```python
from build123d import *

# Parameters (mm, degrees)
F1_DEPTH = 12
F2_R     = 3.5
F4_DEPTH = 4
F6_DEPTH = 4


with BuildPart() as f1:
    # F0 (on Top) → F1 (new body)
    with BuildSketch(Plane.XY):
        with BuildLine():
            Line((10.9868871146, 38.4103373848), (-46.3684160233, 38.4103373848))
            Line((-46.3684160233, 38.4103373848), (-44.9722234273, -1.5713874258))
            ThreePointArc((-44.9722234273, -1.5713874258), (-39.9691757058, -6.4027744503), (-34.9661279843, -1.5713874258))
            Line((-34.9661279843, -1.5713874258), (-36.0131128854, 28.4103373848))
            Line((-36.0131128854, 28.4103373848), (0.9868871146, 28.4103373848))
            Line((0.9868871146, 28.4103373848), (0.9868871146, -26.5896626152))
            ThreePointArc((0.9868871146, -26.5896626152), (35.472835987, -54.4539482888), (55.4723899987, -14.8848072183))
            ThreePointArc((55.4723899987, -14.8848072183), (48.8600464406, -12.3794304662), (46.3546696885, -18.9917740242))
            ThreePointArc((46.3546696885, -18.9917740242), (33.3725030493, -44.6770059472), (10.9868871146, -26.5896626152))
            Line((10.9868871146, -26.5896626152), (10.9868871146, 38.4103373848))
        make_face()
    extrude(amount=F1_DEPTH)

    # F2
    f2_edges = [f1.edges().sort_by_distance(p)[0] for p in [
        (10.986887, 38.410337, 6),
        (-46.368416, 38.410337, 6),
    ]]
    fillet(f2_edges, radius=F2_R)

    # F3 (on face) → F4 (cut)
    with BuildSketch(Plane.XY.offset(12)):
        with BuildLine():
            Line((7.4868871146, 35.16033604), (-42.744059925, 35.16033604))
            ThreePointArc((-42.744059925, 35.16033604), (-42.9238939077, 35.0840010432), (-42.9939062878, 34.9016125575))
            Line((-42.9939062878, 34.9016125575), (-41.7242018955, -1.4579640146))
            ThreePointArc((-41.7242018955, -1.4579640146), (-40.0114090798, -3.1522651845), (-38.219126663, -1.5422839975))
            Line((-38.219126663, -1.5422839975), (-39.3785877977, 31.6603387296))
            Line((-39.3785877977, 31.6603387296), (4.2368884594, 31.6603387296))
            Line((4.2368884594, 31.6603387296), (4.2368884594, -26.5896626152))
            ThreePointArc((4.2368884594, -26.5896626152), (34.7902274998, -51.276440713), (52.5091296718, -16.2195719825))
            ThreePointArc((52.5091296718, -16.2195719825), (50.1948112049, -15.3426907931), (49.3179300155, -17.65700926))
            ThreePointArc((49.3179300155, -17.65700926), (34.0551115365, -47.854513523), (7.7368857699, -26.5896626152))
            Line((7.7368857699, -26.5896626152), (7.7368857699, 34.9103373848))
            ThreePointArc((7.7368857699, 34.9103373848), (7.663662859, 35.0871131292), (7.4868871146, 35.16033604))
        make_face()
    extrude(amount=-F4_DEPTH, mode=Mode.SUBTRACT)

    # F5 (on face) → F6 (cut)
    with BuildSketch(Plane(origin=(0, 0, 0), x_dir=(1, 0, 0), z_dir=(0, 0, -1))):
        with BuildLine():
            Line((-41.7242032033, 1.4579640602), (-42.9939075956, -34.9016125119))
            ThreePointArc((-42.9939075956, -34.9016125119), (-42.923894849, -35.0840019523), (-42.744059925, -35.1603373486))
            Line((-42.744059925, -35.1603373486), (7.4868871146, -35.1603373486))
            ThreePointArc((7.4868871146, -35.1603373486), (7.6636637843, -35.0871140545), (7.7368870784, -34.9103373848))
            Line((7.7368870784, -34.9103373848), (7.7368870784, 26.5896626152))
            ThreePointArc((7.7368870784, 26.5896626152), (34.0551112616, 47.8545122436), (49.3179288223, 17.6570097974))
            ThreePointArc((49.3179288223, 17.6570097974), (50.1948106674, 15.3426896), (52.5091308649, 16.2195714451))
            ThreePointArc((52.5091308649, 16.2195714451), (34.7902277746, 51.2764419924), (4.2368871508, 26.5896626152))
            Line((4.2368871508, 26.5896626152), (4.2368871508, -31.660337421))
            Line((4.2368871508, -31.660337421), (-39.3785864427, -31.660337421))
            Line((-39.3785864427, -31.660337421), (-38.2191253525, 1.5422840291))
            ThreePointArc((-38.2191253525, 1.5422840291), (-40.0114090726, 3.1522664936), (-41.7242032033, 1.4579640602))
        make_face()
    extrude(amount=-F6_DEPTH, mode=Mode.SUBTRACT)


solid = f1.part
```
Check sheet for the modelled part. Datum: model origin and axes. Units: mm. A direction names the side the tool comes from. Coordinates: 2 decimals unless noted, no trailing zeros. Write each loop counter-clockwise with the first axis right and the second up, starting at its lowest first coordinate (ties: lowest second). Pieces come first, ordered by that corner, then holes. Notation, with made-up numbers: (-27, 27) -> (-23, 27) arc R36 cw to (-23, 61) -> close; hole circle Ø6 at (71.25, -10). An arc over 180 degrees is marked (long way). Use a Markdown table: item, result.
1. Sectioned sample at A-A (y = -20.5). Enter the section's corners in (x, z).
Reported:
| item | result |
|---|---|
| outline | (0.99, 0) -> (4.24, 0) -> (4.24, 4) -> (7.74, 4) -> (7.74, 0) -> (10.99, 0) -> (10.99, 12) -> (7.74, 12) -> (7.74, 8) -> (4.24, 8) -> (4.24, 12) -> (0.99, 12) -> close; (46.96, 0) -> (50.37, 0) -> (50.37, 4) -> (53.99, 4) -> (53.99, 0) -> (57.33, 0) -> (57.33, 12) -> (53.99, 12) -> (53.99, 8) -> (50.37, 8) -> (50.37, 12) -> (46.96, 12) -> close |
2. Sectioned sample at D-D (y = 11). Enter the section's corners in (x, z), plus the area to 3 significant figures.
Reported:
| item | result |
|---|---|
| outline | (-45.41, 0) -> (-42.16, 0) -> (-42.16, 4) -> (-38.66, 4) -> (-38.66, 0) -> (-35.41, 0) -> (-35.41, 12) -> (-38.66, 12) -> (-38.66, 8) -> (-42.16, 8) -> (-42.16, 12) -> (-45.41, 12) -> close; (0.99, 0) -> (4.24, 0) -> (4.24, 4) -> (7.74, 4) -> (7.74, 0) -> (10.99, 0) -> (10.99, 12) -> (7.74, 12) -> (7.74, 8) -> (4.24, 8) -> (4.24, 12) -> (0.99, 12) -> close |
| area | 184 mm2 |
3. Tool access check on faces 1 (the flat face through (10.987, 4, 6)), 2 (the flat face through (6, -5, 4)), 3 (the flat face through (0.987, 1, 6)), 4 (the cylindrical face through (33.823, -44.574, 5.916)), 5 (the cylindrical face through (34.584, -47.734, 10.028)). Record the directions out of +Z, -Z, +X, -X, +Y, -Y that give a thin tool (end or side, any length) a straight path to the whole face; none if there is none.
Reported:
| item | result |
|---|---|
| face 1 | +Z, -Z, +Y |
| face 2 | -Z |
| face 3 | +Z, -Z, -Y |
| face 4 | +Z, -Z |
| face 5 | +Z |
4. Scan lines: line 1 along Y through (x, z) = (-22, 10); line 2 along X through (y, z) = (20.5, 1); line 3 along X through (y, z) = (-39.5, 2). Record each from-to range of solid material in increasing order.
Reported:
| item | result |
|---|---|
| line 1 | y = 28.41 to 31.66, 35.16 to 38.41 |
| line 2 | x = -45.74 to -42.49, -38.99 to -35.74, 0.99 to 4.24, 7.74 to 10.99 |
| line 3 | x = 4.08 to 7.79, 11.98 to 16.24, 42.74 to 46.99, 51.19 to 54.9 |
5. Go/stop test with flat-tipped pins: pin 1 Ø4 at (y, z) = (-1.5, 8.5) entering from +X; pin 2 Ø3 at (y, z) = (-20, 9) entering from -X; pin 3 Ø2 at (y, z) = (-7, 9) entering from -X. Record where each tip stops, or that it passes through.
Reported:
| item | result |
|---|---|
| pin 1 | stops at x = 10.99 |
| pin 2 | stops at x = 0.99 |
| pin 3 | stops at x = -41.94 |
6. Sectioned sample at C-C (z = 2.5). Enter the section's corners in (x, y), plus the area to 3 significant figures.
Reported:
| item | result |
|---|---|
| outline | (-46.24, 34.79) -> (-44.97, -1.57) arc R5.01 ccw to (-34.97, -1.57) -> (-36.01, 28.41) -> (0.99, 28.41) -> (0.99, -26.59) arc R28.5 ccw (long way) to (55.47, -14.88) arc R5 ccw to (46.35, -18.99) arc R18.5 cw (long way) to (10.99, -26.59) -> (10.99, 34.91) arc R3.5 ccw to (7.49, 38.41) -> (-42.74, 38.41) arc R3.5 ccw to start; hole (-42.99, 34.9) -> (-41.72, -1.46) arc R1.76 ccw to (-38.22, -1.54) -> (-39.38, 31.66) -> (4.24, 31.66) -> (4.24, -26.59) arc R25.25 ccw (long way) to (52.51, -16.22) arc R1.75 ccw to (49.32, -17.66) arc R21.75 cw (long way) to (7.74, -26.59) -> (7.74, 34.91) arc R0.25 ccw to (7.49, 35.16) -> (-42.74, 35.16) arc R0.25 ccw to start |
| area | 1,530 mm2 |
7. Release check for a two-part mould opening along X. For faces 6 (the cylindrical face through (-45.234, 37.37, 6.084)), 7 (the flat face through (6, -5, 8)) record: pulls with the +X half, pulls with the -X half, needs draft (parallel to the pull), parting line crosses it, or undercut.
Reported:
| item | result |
|---|---|
| face 6 | pulls with the -X half |
| face 7 | undercut |
8. Sectioned sample at B-B (x = -17). Enter the section's corners in (y, z), plus the area to 3 significant figures.
Reported:
| item | result |
|---|---|
| outline | (28.41, 0) -> (31.66, 0) -> (31.66, 4) -> (35.16, 4) -> (35.16, 0) -> (38.41, 0) -> (38.41, 12) -> (35.16, 12) -> (35.16, 8) -> (31.66, 8) -> (31.66, 12) -> (28.41, 12) -> close |
| area | 92.0 mm2 |
